```python
from build123d import *

# Parameters (mm, degrees)
F1_DEPTH = 23
F2_R     = 5
F3_W     = 8
F3_H     = 5
F4_DEPTH = 7


with BuildPart() as f1:
    # F0 (on Front) → F1 (new body)
    with BuildSketch(Plane.XZ):
        with BuildLine():
            ThreePointArc((-20.752427, -5), (-19.287961, -1.464466), (-15.752427, 0))
            Line((-15.752427, 0), (19.247573, 0))
            ThreePointArc((19.247573, 0), (22.783106, -1.464466), (24.247573, -5))
            Line((24.247573, -5), (17.247573, -5))
            Line((17.247573, -5), (17.247573, -8))
            Line((17.247573, -8), (27.247573, -8))
            Line((27.247573, -8), (27.247573, 5))
            Line((27.247573, 5), (-23.752427, 5))
            Line((-23.752427, 5), (-23.752427, -8))
            Line((-23.752427, -8), (-13.752427, -8))
            Line((-13.752427, -8), (-13.752427, -5))
            Line((-13.752427, -5), (-20.752427, -5))
        make_face()
    extrude(amount=F1_DEPTH)

    # F2
    f2_edges = [f1.edges().sort_by_distance(p)[0] for p in [
        (27.247573, -11.5, 5),
        (-23.752427, -11.5, 5),
    ]]
    fillet(f2_edges, radius=F2_R)

    # F3 (on face) → F4 (join)
    with BuildSketch(Plane.XY.offset(5)):
        with Locations((0, -11.5)):
            Rectangle(F3_W, F3_H)
    extrude(amount=F4_DEPTH)


solid = f1.part
```
The model under review builds one solid part; all positions refer to its coordinate system, in mm. A direction names the side the tool comes from. Coordinates: 2 decimals unless noted, no trailing zeros. Write each loop counter-clockwise with the first axis right and the second up, starting at its lowest first coordinate (ties: lowest second). Pieces come first, ordered by that corner, then holes.
1) The part is to be moulded in two halves that separate along Z. For faces 4 (the face through (27.248, -11, -4)), 5 (the face through (22, -11, -8)), 6 (the face through (-19.327, -11.339, -1.504)), say which applies: pulls with the +Z half, pulls with the -Z half, needs draft (parallel to the pull), parting line crosses it, or undercut.
2) We need section D-D on x = 2.5. State the section outline as (y, z) points, then the cut area to 3 significant figures.
3) Clearance check with flat-ended pins moving along their axes: pin 1 Ø4 at (y, z) = (-12, 9) entering from +X; pin 2 Ø5.5 at (x, z) = (1, 8.5) entering from -Y; pin 3 Ø7.5 at (x, y) = (19, -14.5) entering from +Z. State where each tip first meets the part, or that it passes through.
4) We need section A-A on y = -10.25. State the section outline as (x, z) points, then the cut area to 3 significant figures.
5) To check wall thickness, follow probe 1 along X at (y, z) = (-8, -5.75); probe 2 along Z at (x, y) = (-14, -18.5); probe 3 along Z at (x, y) = (15.5, -3.5). State the ranges of each line that lie inside material, in increasing order.
6) We need section B-B on z = -0.75. State the section outline as (x, y) points.
7) We need section C-C on x = 23. State the section outline as (y, z) points, then the cut area to 3 significant figures.
8) Machinability: for faces 1 (the face through (-4, -12, 8)), 2 (the face through (22.744, -11.339, -1.426)), 3 (the face through (0, -9, 8)), which of the approach directions +Z, -Z, +X, -X, +Y, -Y give a long, thin tool a straight path to every point of the face, cutting with its end or side? Answer none if there is none.
Answer list:
1. face 4: needs draft
1. face 5: pulls with the -Z half
1. face 6: undercut
2. outline: (-23, 0) - (0, 0) - (0, 5) - (-9, 5) - (-9, 12) - (-14, 12) - (-14, 5) - (-23, 5) - close
2. area: 150 mm2
3. pin 1: stops at x = 4
3. pin 2: stops at y = -14
3. pin 3: stops at z = 5
4. outline: (-23.75, -8) - (-13.75, -8) - (-13.75, -5) - (-20.75, -5) arc R5 cw to (-15.75, 0) - (19.25, 0) arc R5 cw to (24.25, -5) - (17.25, -5) - (17.25, -8) - (27.25, -8) - (27.25, 0) arc R5 ccw to (22.25, 5) - (4, 5) - (4, 12) - (-4, 12) - (-4, 5) - (-18.75, 5) arc R5 ccw to (-23.75, 0) - close
4. area: 401 mm2
5. probe 1: x = -23.75 to -13.75, 17.25 to 27.25
5. probe 2: z = -8 to -5, 0 to 5
5. probe 3: z = 0 to 5
6. outline: (-23.75, -23) - (-18.39, -23) - (-18.39, 0) - (-23.75, 0) - close; (21.88, -23) - (27.25, -23) - (27.25, 0) - (21.88, 0) - close
7. outline: (-23, -8) - (0, -8) - (0, -5) - (-23, -5) - close; (-23, -1.7) - (0, -1.7) - (0, 4.94) - (-23, 4.94) - close
7. area: 222 mm2
8. face 1: +Z, -X, +Y, -Y
8. face 2: +Y, -Y
8. face 3: +Z, +X, -X, +Y
